from build123d import *

# Parameters (mm, degrees)
SKETCH_2_R      = 1.6
SKETCH_2_W      = 3
SKETCH_2_H      = 40
SKETCH_2_H_2    = 45
SKETCH_2_R_2    = 3
EXTRUDE_1_DEPTH = 3
FILLET_1_R      = 15


with BuildPart() as part:
    # 草图2 → 凸台-拉伸1 (new body)
    with BuildSketch(Plane(origin=(0, 0, 0), x_dir=(1, 0, 0), z_dir=(0, 1, 0))):
        Polygon((100, -68.942911166), (100, 68.942911166), (-100, 68.942911166), (-100, -68.942911166), (0, -68.942911166), align=None)
        with Locations(Location((-52.5, -52.5, 0), (0, 0, 270))):
            Circle(SKETCH_2_R, mode=Mode.SUBTRACT)
        with Locations((-87.942911166, -40)):
            Rectangle(SKETCH_2_W, SKETCH_2_H, mode=Mode.SUBTRACT)
        with Locations((-74.942911166, -40)):
            Rectangle(SKETCH_2_W, SKETCH_2_H, mode=Mode.SUBTRACT)
        with Locations(Location((-45.428932188, -45.428932188, 0), (0, 0, 270))):
            Circle(SKETCH_2_R, mode=Mode.SUBTRACT)
        with Locations(Location((-38.357864376, -38.357864376, 0), (0, 0, 270))):
            Circle(SKETCH_2_R, mode=Mode.SUBTRACT)
        with BuildLine():
            ThreePointArc((22.714466094, -53.428932188), (26.714466094, -57.428932188), (22.714466094, -61.428932188))
            Line((22.714466094, -61.428932188), (-22.714466094, -61.428932188))
            ThreePointArc((-22.714466094, -61.428932188), (-26.714466094, -57.428932188), (-22.714466094, -53.428932188))
            Line((-22.714466094, -53.428932188), (22.714466094, -53.428932188))
        make_face(mode=Mode.SUBTRACT)
        with BuildLine():
            Line((22.714466094, -46.428932188), (-22.714466094, -46.428932188))
            ThreePointArc((-22.714466094, -46.428932188), (-26.714466094, -42.428932188), (-22.714466094, -38.428932188))
            Line((-22.714466094, -38.428932188), (22.714466094, -38.428932188))
            ThreePointArc((22.714466094, -38.428932188), (26.714466094, -42.428932188), (22.714466094, -46.428932188))
        make_face(mode=Mode.SUBTRACT)
        with Locations(Location((38.357864376, -38.357864376, 0), (0, 0, 270))):
            Circle(SKETCH_2_R, mode=Mode.SUBTRACT)
        with Locations(Location((52.5, -52.5, 0), (0, 0, 270))):
            Circle(SKETCH_2_R, mode=Mode.SUBTRACT)
        with Locations(Location((45.428932188, -45.428932188, 0), (0, 0, 270))):
            Circle(SKETCH_2_R, mode=Mode.SUBTRACT)
        with Locations((74.942911166, -42.5)):
            Rectangle(SKETCH_2_W, SKETCH_2_H_2, mode=Mode.SUBTRACT)
        with Locations((87.942911166, -42.5)):
            Rectangle(SKETCH_2_W, SKETCH_2_H_2, mode=Mode.SUBTRACT)
        with BuildLine():
            Line((22.714466094, -31.428932188), (-22.714466094, -31.428932188))
            ThreePointArc((-22.714466094, -31.428932188), (-26.714466094, -27.428932188), (-22.714466094, -23.428932188))
            Line((-22.714466094, -23.428932188), (22.714466094, -23.428932188))
            ThreePointArc((22.714466094, -23.428932188), (26.714466094, -27.428932188), (22.714466094, -31.428932188))
        make_face(mode=Mode.SUBTRACT)
        with BuildLine():
            ThreePointArc((-62.5, -32.5), (-65, -35), (-67.5, -32.5))
            Line((-67.5, -32.5), (-67.5, 32.5))
            ThreePointArc((-67.5, 32.5), (-65, 35), (-62.5, 32.5))
            Line((-62.5, 32.5), (-62.5, -32.5))
        make_face(mode=Mode.SUBTRACT)
        with BuildLine():
            ThreePointArc((-57.5, 27.5), (-55, 30), (-52.5, 27.5))
            Line((-52.5, 27.5), (-52.5, -27.5))
            ThreePointArc((-52.5, -27.5), (-55, -30), (-57.5, -27.5))
            Line((-57.5, -27.5), (-57.5, 27.5))
        make_face(mode=Mode.SUBTRACT)
        with BuildLine():
            Line((-47.5, -22.5), (-47.5, 22.5))
            ThreePointArc((-47.5, 22.5), (-45, 25), (-42.5, 22.5))
            Line((-42.5, 22.5), (-42.5, -22.5))
            ThreePointArc((-42.5, -22.5), (-45, -25), (-47.5, -22.5))
        make_face(mode=Mode.SUBTRACT)
        with BuildLine():
            Line((-37.5, -17.5), (-37.5, 17.5))
            ThreePointArc((-37.5, 17.5), (-35, 20), (-32.5, 17.5))
            Line((-32.5, 17.5), (-32.5, -17.5))
            ThreePointArc((-32.5, -17.5), (-35, -20), (-37.5, -17.5))
        make_face(mode=Mode.SUBTRACT)
        with BuildLine():
            Line((-27.5, -12.5), (-27.5, 12.5))
            ThreePointArc((-27.5, 12.5), (-25, 15), (-22.5, 12.5))
            Line((-22.5, 12.5), (-22.5, -12.5))
            ThreePointArc((-22.5, -12.5), (-25, -15), (-27.5, -12.5))
        make_face(mode=Mode.SUBTRACT)
        with Locations(Location((0, 0, 0), (0, 0, 270))):
            Circle(SKETCH_2_R_2, mode=Mode.SUBTRACT)
        with BuildLine():
            Line((22.714466094, 23.428932188), (-22.714466094, 23.428932188))
            ThreePointArc((-22.714466094, 23.428932188), (-26.714466094, 27.428932188), (-22.714466094, 31.428932188))
            Line((-22.714466094, 31.428932188), (22.714466094, 31.428932188))
            ThreePointArc((22.714466094, 31.428932188), (26.714466094, 27.428932188), (22.714466094, 23.428932188))
        make_face(mode=Mode.SUBTRACT)
        with Locations((-87.942911166, 40)):
            Rectangle(SKETCH_2_W, SKETCH_2_H, mode=Mode.SUBTRACT)
        with Locations((-74.942911166, 40)):
            Rectangle(SKETCH_2_W, SKETCH_2_H, mode=Mode.SUBTRACT)
        with Locations(Location((-45.428932188, 45.428932188, 0), (0, 0, 270))):
            Circle(SKETCH_2_R, mode=Mode.SUBTRACT)
        with Locations(Location((-52.5, 52.5, 0), (0, 0, 270))):
            Circle(SKETCH_2_R, mode=Mode.SUBTRACT)
        with Locations(Location((-38.357864376, 38.357864376, 0), (0, 0, 270))):
            Circle(SKETCH_2_R, mode=Mode.SUBTRACT)
        with BuildLine():
            ThreePointArc((-22.714466094, 38.428932188), (-26.456123481, 41.014718626), (-25.360217405, 45.428932188))
            ThreePointArc((-25.360217405, 45.428932188), (-24.128679656, 46.170589575), (-22.714466094, 46.428932188))
            Line((-22.714466094, 46.428932188), (22.714466094, 46.428932188))
            ThreePointArc((22.714466094, 46.428932188), (26.714466094, 42.428932188), (22.714466094, 38.428932188))
            Line((22.714466094, 38.428932188), (-22.714466094, 38.428932188))
        make_face(mode=Mode.SUBTRACT)
        with BuildLine():
            ThreePointArc((22.714466094, 61.428932188), (26.714466094, 57.428932188), (22.714466094, 53.428932188))
            Line((22.714466094, 53.428932188), (-22.714466094, 53.428932188))
            ThreePointArc((-22.714466094, 53.428932188), (-26.714466094, 57.428932188), (-22.714466094, 61.428932188))
            Line((-22.714466094, 61.428932188), (22.714466094, 61.428932188))
        make_face(mode=Mode.SUBTRACT)
        with BuildLine():
            Line((22.5, -12.5), (22.5, 12.5))
            ThreePointArc((22.5, 12.5), (25, 15), (27.5, 12.5))
            Line((27.5, 12.5), (27.5, -12.5))
            ThreePointArc((27.5, -12.5), (25, -15), (22.5, -12.5))
        make_face(mode=Mode.SUBTRACT)
        with BuildLine():
            Line((32.5, -17.5), (32.5, 17.5))
            ThreePointArc((32.5, 17.5), (35, 20), (37.5, 17.5))
            Line((37.5, 17.5), (37.5, -17.5))
            ThreePointArc((37.5, -17.5), (35, -20), (32.5, -17.5))
        make_face(mode=Mode.SUBTRACT)
        with BuildLine():
            Line((42.5, -22.5), (42.5, 22.5))
            ThreePointArc((42.5, 22.5), (45, 25), (47.5, 22.5))
            Line((47.5, 22.5), (47.5, -22.5))
            ThreePointArc((47.5, -22.5), (45, -25), (42.5, -22.5))
        make_face(mode=Mode.SUBTRACT)
        with BuildLine():
            Line((52.5, -27.5), (52.5, 27.5))
            ThreePointArc((52.5, 27.5), (55, 30), (57.5, 27.5))
            Line((57.5, 27.5), (57.5, -27.5))
            ThreePointArc((57.5, -27.5), (55, -30), (52.5, -27.5))
        make_face(mode=Mode.SUBTRACT)
        with BuildLine():
            Line((62.5, -32.5), (62.5, 32.5))
            ThreePointArc((62.5, 32.5), (65, 35), (67.5, 32.5))
            Line((67.5, 32.5), (67.5, -32.5))
            ThreePointArc((67.5, -32.5), (65, -35), (62.5, -32.5))
        make_face(mode=Mode.SUBTRACT)
        with Locations(Location((38.357864376, 38.357864376, 0), (0, 0, 270))):
            Circle(SKETCH_2_R, mode=Mode.SUBTRACT)
        with Locations(Location((45.428932188, 45.428932188, 0), (0, 0, 270))):
            Circle(SKETCH_2_R, mode=Mode.SUBTRACT)
        with Locations((74.942911166, 40)):
            Rectangle(SKETCH_2_W, SKETCH_2_H, mode=Mode.SUBTRACT)
        with Locations((87.942911166, 40)):
            Rectangle(SKETCH_2_W, SKETCH_2_H, mode=Mode.SUBTRACT)
        with Locations(Location((52.5, 52.5, 0), (0, 0, 270))):
            Circle(SKETCH_2_R, mode=Mode.SUBTRACT)
    extrude(amount=EXTRUDE_1_DEPTH)

    # 圆角1
    fillet_1_edges = [part.edges().sort_by_distance(p)[0] for p in [
        (-100, 1.5, -68.942911166),
        (100, 1.5, -68.942911166),
        (100, 1.5, 68.942911166),
        (-100, 1.5, 68.942911166),
    ]]
    fillet(fillet_1_edges, radius=FILLET_1_R)


solid = part.part
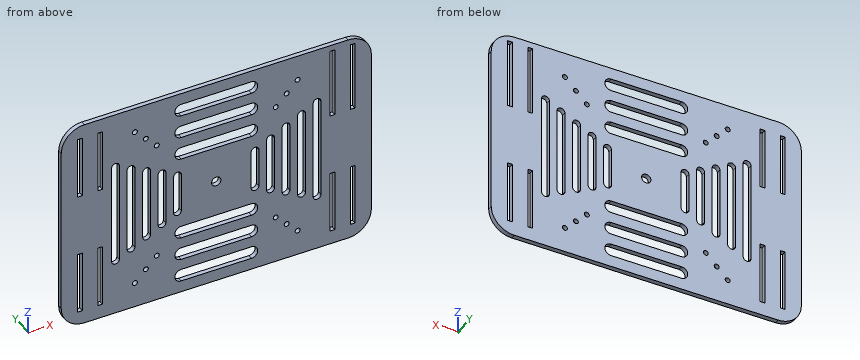
Build history of the part. All positions in model axes, mm. Round coordinates to 2 decimals unless told otherwise and drop trailing zeros. Write each loop counter-clockwise with the first axis right and the second up, starting at its lowest first coordinate (ties: lowest second). Pieces come first, ordered by that corner, then holes. Notation, with made-up numbers: M -23,-30 L 7,-30 A30 ccw 7,7 Z; hole C 4.5,20 d5. An arc over 180 degrees is marked long. Answer in a Markdown table with one row per item.
1. Saw through at A-A (x = 17). List the corners of the cut face in (y, z).
Geometry check:
| item | result |
|---|---|
| outline | M 0,-68.94 L 3,-68.94 L 3,-61.43 L 0,-61.43 Z; M 0,-53.43 L 3,-53.43 L 3,-46.43 L 0,-46.43 Z; M 0,-38.43 L 3,-38.43 L 3,-31.43 L 0,-31.43 Z; M 0,-23.43 L 3,-23.43 L 3,23.43 L 0,23.43 Z; M 0,31.43 L 3,31.43 L 3,38.43 L 0,38.43 Z; M 0,46.43 L 3,46.43 L 3,53.43 L 0,53.43 Z; M 0,61.43 L 3,61.43 L 3,68.94 L 0,68.94 Z |
2. Saw through at B-B (z = 58). List the corners of the cut face in (x, y), and give its area (3 significant figures).
Geometry check:
| item | result |
|---|---|
| outline | M -99.44,0 L -89.44,0 L -89.44,3 L -99.44,3 Z; M -86.44,0 L -76.44,0 L -76.44,3 L -86.44,3 Z; M -73.44,0 L -26.67,0 L -26.67,3 L -73.44,3 Z; M 26.67,0 L 73.44,0 L 73.44,3 L 26.67,3 Z; M 76.44,0 L 86.44,0 L 86.44,3 L 76.44,3 Z; M 89.44,0 L 99.44,0 L 99.44,3 L 89.44,3 Z |
| area | 401 mm2 |
3. Saw through at C-C (z = 0). State how many separate pieces and enclosed holes the cut face has, and give its area (3 significant figures).
Geometry check:
| item | result |
|---|---|
| separate pieces | 12 |
| enclosed holes | 0 |
| area | 432 mm2 |
4. Flat gauge pin, fed straight in: P1, Ø0.9, axis at x = 88, y = 1, coming from the -Z side. Where does the tip first touch, or does it go through?
Geometry check:
| item | result |
|---|---|
| P1 | z = -68.72 |
5. Probe L1, parallel to Z at x = -37, y = 2.35; L2, parallel to Z at x = -39.5, y = 1.5; L3, parallel to X at y = 1.2, z = 63. List the from-to ranges inside material, lowest first. Write a range as [from, to].
Geometry check:
| item | result |
|---|---|
| L1 | [-68.94, -39.2], [-37.51, -19], [19, 37.51], [39.2, 68.94] |
| L2 | [-68.94, -39.48], [-37.24, 37.24], [39.48, 68.94] |
| L3 | [-96.96, 73.44], [76.44, 86.44], [89.44, 96.96] |
